```python
from build123d import *

# Parameters (mm, degrees)
SKETCH_1_W             = 29
SKETCH_1_H             = 29
EXTRUDE_1_DEPTH        = 2
FILLET_1_R             = 1
HOLE_WIZARD_M3_1_D     = 3.4
HOLE_WIZARD_M3_1_DEPTH = 7.5
HOLE_WIZARD_M3_1_TIP   = 1.021463052
SKETCH_4_R             = 10
CUT_EXTRUDE_1_DEPTH    = 21.603397778


with BuildPart() as part:
    # 草图1 → 凸台-拉伸1 (new body)
    with BuildSketch(Plane.XY):
        Rectangle(SKETCH_1_W, SKETCH_1_H)
    extrude(amount=EXTRUDE_1_DEPTH)

    # 圆角1
    fillet_1_edges = [part.edges().sort_by_distance(p)[0] for p in [
        (14.5, -14.5, 1),
        (-14.5, -14.5, 1),
        (-14.5, 14.5, 1),
        (14.5, 14.5, 1),
    ]]
    fillet(fillet_1_edges, radius=FILLET_1_R)

    # M3 间隙孔1
    with Locations(Plane.XY.offset(2)):
        with Locations((-11, 11), (11, 11), (-11, -11), (11, -11)):
            Hole(HOLE_WIZARD_M3_1_D / 2, depth=HOLE_WIZARD_M3_1_DEPTH)
            with Locations((0, 0, -(HOLE_WIZARD_M3_1_DEPTH + HOLE_WIZARD_M3_1_TIP / 2))):  # 118° drill point
                Cone(0, HOLE_WIZARD_M3_1_D / 2, HOLE_WIZARD_M3_1_TIP, mode=Mode.SUBTRACT)

    # 草图4 → 切除-拉伸1 (cut, through all)
    with BuildSketch(Plane.XY.offset(2)):
        Circle(SKETCH_4_R)
    extrude(amount=-CUT_EXTRUDE_1_DEPTH, mode=Mode.SUBTRACT)


solid = part.part
```
Could you check a few things on this model? Use its own coordinates, in mm. Coordinates: 2 decimals unless noted, no trailing zeros. Write each loop counter-clockwise with the first axis right and the second up, starting at its lowest first coordinate (ties: lowest second). Pieces come first, ordered by that corner, then holes. Notation, with made-up numbers: (-36.75, 66) -> (-18.75, 66) arc R8 ccw to (-18.75, 70) -> close; hole circle Ø6 at (89.25, 75). An arc over 180 degrees is marked (long way). One line per question, with ' | ' between items. Start each with the question number.
1. If we section it at D-D (y = 0): Please give me the cut outline in (x, z), and give its area (3 significant figures).
2. If we section it at A-A (y = -11): Please give me the cut outline in (x, z).
3. Please list where these lines run through material, in increasing order: line 1 along Y through (x, z) = (11, 1.1); line 2 along X through (y, z) = (0.25, 0.8); line 3 along X through (y, z) = (11.75, 1.35).
4. Thinking about a two-plate mould opening in Y: for faces 1 (the face through (0, 14.5, 1)), 2 (the face through (0, -14.5, 1)), 3 (the face through (-12.62, 11.51, 0.99)), which applies, pulls with the +Y half, pulls with the -Y half, needs draft (parallel to the pull), parting line crosses it, or undercut?
5. If we section it at B-B (z = 1.25): Please give me the cut outline in (x, y).
Return value:
1) outline: (-14.5, 0) -> (-10, 0) -> (-10, 2) -> (-14.5, 2) -> close; (10, 0) -> (14.5, 0) -> (14.5, 2) -> (10, 2) -> close | area: 18.0 mm²
2) outline: (-14.5, 0) -> (-12.7, 0) -> (-12.7, 2) -> (-14.5, 2) -> close; (-9.3, 0) -> (9.3, 0) -> (9.3, 2) -> (-9.3, 2) -> close; (12.7, 0) -> (14.5, 0) -> (14.5, 2) -> (12.7, 2) -> close
3) line 1: y = -14.5 to -12.7, -9.3 to 9.3, 12.7 to 14.5 | line 2: x = -14.5 to -10, 10 to 14.5 | line 3: x = -14.5 to -12.53, -9.47 to 9.47, 12.53 to 14.5
4) face 1: pulls with the +Y half | face 2: pulls with the -Y half | face 3: undercut
5) outline: (-14.5, -13.5) arc R1 ccw to (-13.5, -14.5) -> (13.5, -14.5) arc R1 ccw to (14.5, -13.5) -> (14.5, 13.5) arc R1 ccw to (13.5, 14.5) -> (-13.5, 14.5) arc R1 ccw to (-14.5, 13.5) -> close; hole circle Ø3.4 at (-11, -11); hole circle Ø3.4 at (-11, 11); hole circle Ø20 at (0, 0); hole circle Ø3.4 at (11, -11); hole circle Ø3.4 at (11, 11)
